For this review, take the finished solid that the model builds, in its own axes (mm). Coordinates: 2 decimals unless noted, no trailing zeros. Write each loop counter-clockwise with the first axis right and the second up, starting at its lowest first coordinate (ties: lowest second). Pieces come first, ordered by that corner, then holes.
```python
from build123d import *

# Parameters (mm, degrees)
SKETCH_R          = 14.9
SKETCH_R_2        = 2.55
PAD_DEPTH         = 10.5
FILLET_R          = 0.5
SKETCH001_R       = 0.35
PAD001_DEPTH      = 5.25
PAD001_DEPTH_BACK = 3.5


with BuildPart() as fillet_body:
    # Sketch → Pad (new body)
    with BuildSketch(Plane.XY.offset(0.1)):
        with Locations((14.25, 0)):
            Circle(SKETCH_R)
        with Locations((14.25, 0)):
            Circle(SKETCH_R_2, mode=Mode.SUBTRACT)
    extrude(amount=PAD_DEPTH)

    # Fillet
    fillet_edges = [fillet_body.edges().sort_by_distance(p)[0] for p in [
        (11.7, 0, 10.6),
        (-0.65, 0, 10.6),
        (-0.65, 0, 0.1),
    ]]
    fillet(fillet_edges, radius=FILLET_R)


with BuildPart() as obj1:
    # Sketch001 → Pad001 (new body, two sides)
    with BuildSketch(Plane.XY.offset(0.5)) as pad001_sk:
        Circle(SKETCH001_R)
        with Locations((28.5, 0)):
            Circle(SKETCH001_R)
    extrude(amount=PAD001_DEPTH)
    extrude(pad001_sk.sketch, amount=-PAD001_DEPTH_BACK)

    # obj1: union Fillet body
    add(fillet_body.part)


solid = obj1.part
```
1) The part is to be moulded in two halves that separate along Y. For faces 1 (the face through (17, 0, 0.1)), 2 (the face through (11.7, 0.1, 5)), 3 (the face through (3.27, 10.07, 5.28)), say which applies: pulls with the +Y half, pulls with the -Y half, needs draft (parallel to the pull), parting line crosses it, or undercut.
2) For L1, parallel to Y at x = 14.25, z = 2.5; L2, parallel to Z at x = 24.75, y = -5; L3, parallel to X at y = -0.5, z = 9, list the stretches that pass through material, from the lowest coordinate up.
3) Consider section A-A (x = 14.25). Give the boundary of the cut face in (y, z), then the cut area to 3 significant figures.
4) Consider section C-C (z = -0.5). Give the boundary of the cut face in (x, y), then the cut area to 3 significant figures.
5) Consider section B-B (z = 7). Give the boundary of the cut face in (x, y).
6) Clearance check with flat-ended pins moving along their axes: P1, Ø8.5, axis at x = 17, y = -0.5, coming from the -Z side; P2, Ø4, axis at x = 2.5, z = 3, coming from the +Y side; P3, Ø6, axis at x = 21.5, z = -1, coming from the +Y side. State where each tip first meets the part, or that it passes through.
Results:
1. face 1: needs draft
1. face 2: undercut
1. face 3: parting line crosses it
2. L1: y = -14.9 to -2.55, 2.55 to 14.9
2. L2: z = 0.1 to 10.6
2. L3: x = -0.64 to 11.75, 16.75 to 29.14
3. outline: (-14.9, 0.6) arc R0.5 ccw to (-14.4, 0.1) - (-2.55, 0.1) - (-2.55, 10.1) arc R0.5 ccw to (-3.05, 10.6) - (-14.4, 10.6) arc R0.5 ccw to (-14.9, 10.1) - close; (2.55, 0.1) - (14.4, 0.1) arc R0.5 ccw to (14.9, 0.6) - (14.9, 10.1) arc R0.5 ccw to (14.4, 10.6) - (3.05, 10.6) arc R0.5 ccw to (2.55, 10.1) - close
3. area: 259 mm2
4. outline: circle Ø0.7 at (0, 0); circle Ø0.7 at (28.5, 0)
4. area: 0.770 mm2
5. outline: circle Ø29.8 at (14.25, 0); hole circle Ø5.1 at (14.25, 0)
6. P1: stops at z = 0.1
6. P2: stops at y = 11.27
6. P3: stops at y = 14.14
